Geometry check sheet. Reference: the model listing, model coordinates, mm. Round coordinates to 2 decimals unless told otherwise and drop trailing zeros. Order: outer loops, then holes, each group sorted by start corner. A loop starts at its lowest first (then second) coordinate and runs counter-clockwise, first axis right, second up.
(1) Sectioned sample at C-C (x = 14). Record the boundary of the cut face in (y, z), plus the area to 3 significant figures.
(2) Sectioned sample at D-D (x = 35). Give the number of separate pieces and of enclosed holes in the cut face, plus the area to 3 significant figures.
(3) Material ranges on line 1 along Y through (x, z) = (18, 0); line 2 along Y through (x, z) = (37, 0); line 3 along Y through (x, z) = (25.5, 0), recorded low to high.
(4) Go/stop test with flat-tipped pins: pin 1 (5 mm diameter, centred on x = 40.5, y = 9, fed in from +Z); pin 2 (4 mm diameter, centred on x = 29.5, z = 28, fed in from +Y); pin 3 (5 mm diameter, centred on x = 27.5, z = -15, fed in from +Y). Record where each tip stops, or that it passes through.
(5) Sectioned sample at B-B (z = 0). Record the boundary of the cut face in (x, y), plus the area to 3 significant figures.
(6) Sectioned sample at A-A (y = 0). Record the boundary of the cut face in (x, z), plus the area to 4 significant figures.
from build123d import *

# Parameters (mm, degrees)
SKIZZE1_R                           = 50
SKIZZE1_R_2                         = 2.5
AUFSATZ_LINEAR_AUSTRAGEN1_DEPTH     = 50
FASE1_SIZE                          = 25
F_4_0_4_DURCHMESSER_BOHRUNG1_REACH  = 90.388
F_4_0_4_DURCHMESSER_BOHRUNG1_BORE_R = 2


with BuildPart() as part:
    # Skizze1 → Aufsatz-Linear austragen1 (new body)
    with BuildSketch(Plane(origin=(0, 0, 0), x_dir=(0, 0, -1), z_dir=(1, 0, 0))):
        Circle(SKIZZE1_R)
        Circle(SKIZZE1_R_2, mode=Mode.SUBTRACT)
    extrude(amount=AUFSATZ_LINEAR_AUSTRAGEN1_DEPTH)

    # Fase1
    fase1_edges = [part.edges().sort_by_distance(p)[0] for p in [
        (50, 0, 50),
    ]]
    chamfer(fase1_edges, length=FASE1_SIZE)

    # Ø4.0 (4) Durchmesser Bohrung1 bore (on position points) → Ø4.0 (4) Durchmesser Bohrung1 (cut, up to next)
    with BuildSketch(Plane(origin=(47, 28, 0), x_dir=(0.707106781, -0.707106781, 0), z_dir=(0.707106781, 0.707106781, 0)), mode=Mode.PRIVATE) as f_4_0_4_durchmesser_bohrung1_sk1:
        Circle(F_4_0_4_DURCHMESSER_BOHRUNG1_BORE_R)
    f_4_0_4_durchmesser_bohrung1_tool1 = extrude(f_4_0_4_durchmesser_bohrung1_sk1.sketch, amount=-F_4_0_4_DURCHMESSER_BOHRUNG1_REACH, mode=Mode.PRIVATE) & part.part
    add(f_4_0_4_durchmesser_bohrung1_tool1.solids().sort_by_distance((47, 28, 0))[0], mode=Mode.SUBTRACT)


solid = part.part
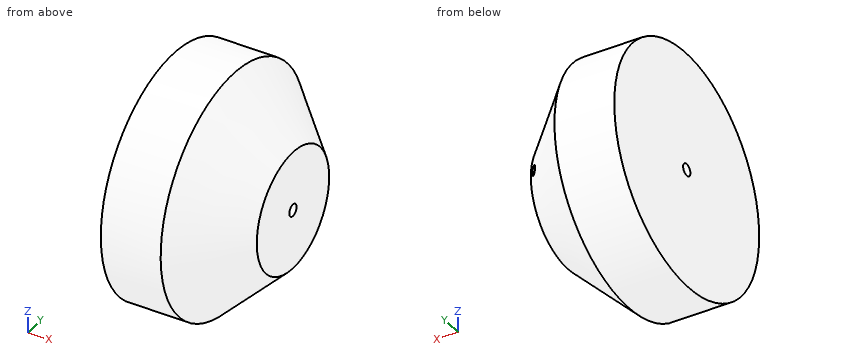
Answer below:
1. outline: circle Ø100 at (0, 0); hole circle Ø5 at (0, 0)
1. area: 7,830 mm2
2. separate pieces: 1
2. enclosed holes: 2
2. area: 4,990 mm2
3. line 1: y = -50 to -2.5, 2.5 to 50
3. line 2: y = -38 to -2.5, 2.5 to 15.17, 20.83 to 38
3. line 3: y = -49.5 to -2.5, 2.5 to 3.67, 9.33 to 49.5
4. pin 1: stops at z = 35.96
4. pin 2: stops at y = 38.75
4. pin 3: stops at y = 47.81
5. outline: (0, -50) - (25, -50) - (50, -25) - (50, -2.5) - (0, -2.5) - close; (0, 2.5) - (18.67, 2.5) - (45.59, 29.41) - (25, 50) - (0, 50) - close; (24.33, 2.5) - (50, 2.5) - (50, 25) - (48.41, 26.59) - close
5. area: 3,980 mm2
6. outline: (0, -50) - (25, -50) - (50, -25) - (50, -2.5) - (0, -2.5) - close; (0, 2.5) - (50, 2.5) - (50, 25) - (25, 50) - (0, 50) - close
6. area: 4,125 mm2
